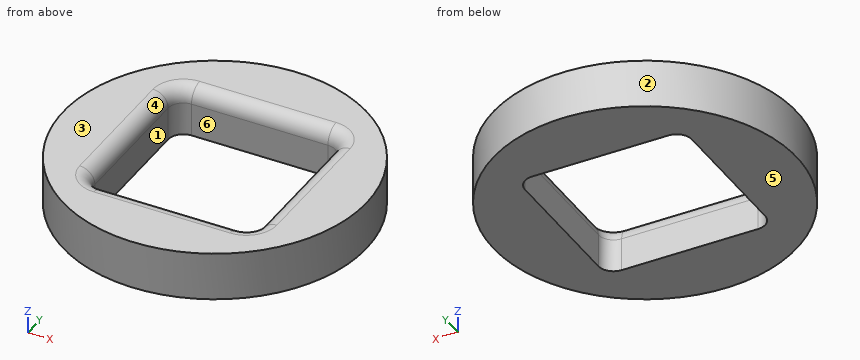
from build123d import *

# Parameters (mm, degrees)
SKETCH1_R               = 25
SKETCH1_W               = 27.5
SKETCH1_H               = 27.5
BOSS_EXTRUDE1_DEPTH     = 55
BOSS_EXTRUDE2_START     = 5
SKETCH2_R               = 25
SKETCH2_W               = 27.5
SKETCH2_H               = 27.5
BOSS_EXTRUDE2_DEPTH     = 5
SKETCH3_W               = 25
SKETCH3_H               = 50
BOSS_EXTRUDE3_DEPTH     = 80
FILLET1_R               = 2.5
FILLET2_R               = 2.5
SKETCH21_W              = 54.3
SKETCH21_H              = 20.3
CUT_EXTRUDE1_DEPTH      = 11.3
SKETCH22_W              = 40.3
SKETCH22_H              = 20.3
CUT_EXTRUDE2_DEPTH      = 93.059763198
CUT_EXTRUDE3_DEPTH      = 88.464278423
SKETCH23_R              = 2.15
CUT_EXTRUDE4_DEPTH      = 93.059763198
CUT_EXTRUDE7_DEPTH      = 27.5
CUT_EXTRUDE8_DEPTH      = 93.059763198
CUT_EXTRUDE8_DEPTH_BACK = 93.059763198
SKETCH25_W              = 132
SKETCH25_H              = 50


with BuildPart() as part:
    # Sketch1 → Boss-Extrude1 (new body)
    with BuildSketch(Plane.XY):
        Circle(SKETCH1_R)
        Rectangle(SKETCH1_W, SKETCH1_H, mode=Mode.SUBTRACT)
    extrude(amount=BOSS_EXTRUDE1_DEPTH)

    # Sketch2 → Boss-Extrude2 (add)
    # profile 1 of 2: a face of its own
    with BuildSketch(Plane(origin=(0, 0, 0), x_dir=(-1, 0, 0), z_dir=(0, 0, -1)).offset(BOSS_EXTRUDE2_START)):
        Circle(SKETCH2_R)
        Rectangle(SKETCH2_W, SKETCH2_H, mode=Mode.SUBTRACT)
    # profile 2 of 2: a face of its own
    with BuildSketch(Plane(origin=(0, 0, 0), x_dir=(-1, 0, 0), z_dir=(0, 0, -1)).offset(BOSS_EXTRUDE2_START)):
        Rectangle(SKETCH2_W, SKETCH2_H)
    extrude(amount=-BOSS_EXTRUDE2_DEPTH)

    # Sketch3 → Boss-Extrude3 (add)
    with BuildSketch(Plane(origin=(0, 0, -5), x_dir=(-1, 0, 0), z_dir=(0, 0, -1))):
        with Locations((12.5, 0)):
            Rectangle(SKETCH3_W, SKETCH3_H)
    extrude(amount=BOSS_EXTRUDE3_DEPTH)

    # Fillet1
    fillet1_edges = [part.edges().sort_by_distance(p)[0] for p in [
        (-13.75, 13.75, 27.5),
        (-13.75, -13.75, 27.5),
        (13.75, -13.75, 27.5),
        (13.75, 13.75, 27.5),
    ]]
    fillet(fillet1_edges, radius=FILLET1_R)

    # Fillet2
    fillet2_edges = [part.edges().sort_by_distance(p)[0] for p in [
        (0, 13.75, 55),
        (-13.75, 0, 55),
        (0, -13.75, 55),
        (13.75, 0, 55),
        (-13.017766953, 13.017766953, 55),
        (-13.017766953, -13.017766953, 55),
        (13.017766953, -13.017766953, 55),
        (13.017766953, 13.017766953, 55),
    ]]
    fillet(fillet2_edges, radius=FILLET2_R)

    # Sketch21 → Cut-Extrude1 (cut)
    with BuildSketch(Plane(origin=(0, 0, 0), x_dir=(0, 0, -1), z_dir=(1, 0, 0))):
        with Locations((51.85, 0)):
            Rectangle(SKETCH21_W, SKETCH21_H)
    extrude(amount=-CUT_EXTRUDE1_DEPTH, mode=Mode.SUBTRACT)

    # Sketch22 → Cut-Extrude2 (cut, through all)
    with BuildSketch(Plane(origin=(0, 0, 0), x_dir=(0, 0, -1), z_dir=(1, 0, 0))):
        with Locations((51.7, 0)):
            Rectangle(SKETCH22_W, SKETCH22_H)
    extrude(amount=-CUT_EXTRUDE2_DEPTH, mode=Mode.SUBTRACT)

    # Sketch18 → Cut-Extrude3 (cut, through all)
    with BuildSketch(Plane.XY.offset(-5)):
        with BuildLine():
            Line((-25, -25), (0, -25))
            ThreePointArc((0, -25), (-17.67766953, -17.67766953), (-25, 0))
            Line((-25, 0), (-25, -25))
        make_face()
        with BuildLine():
            Line((-25, 25), (-25, 0))
            ThreePointArc((-25, 0), (-17.67766953, 17.67766953), (0, 25))
            Line((0, 25), (-25, 25))
        make_face()
    extrude(amount=-CUT_EXTRUDE3_DEPTH, mode=Mode.SUBTRACT)

    # Sketch23 → Cut-Extrude4 (cut, through all)
    with BuildSketch(Plane(origin=(0, 0, 0), x_dir=(0, 0, -1), z_dir=(1, 0, 0))):
        with Locations(Location((27.85, -5.25, 0), (0, 0, 90))):
            Circle(SKETCH23_R)
        with Locations(Location((75.85, 5.25, 0), (0, 0, 90))):
            Circle(SKETCH23_R)
        with Locations(Location((75.85, -5.25, 0), (0, 0, 90))):
            Circle(SKETCH23_R)
        with Locations(Location((27.85, 5.25, 0), (0, 0, 90))):
            Circle(SKETCH23_R)
    extrude(amount=-CUT_EXTRUDE4_DEPTH, mode=Mode.SUBTRACT)

    # Sketch24 → Cut-Extrude7 (cut, symmetric)
    with BuildSketch(Plane(origin=(0, 0, -51.7), x_dir=(-1, 0, 0), z_dir=(0, 0, -1))):
        with BuildLine():
            Line((13.3, 10.15), (13.3, -10.15))
            Line((13.3, -10.15), (22.846826913, -10.15))
            ThreePointArc((22.846826913, -10.15), (25, 0), (22.846826913, 10.15))
            Line((22.846826913, 10.15), (13.3, 10.15))
        make_face()
    extrude(amount=CUT_EXTRUDE7_DEPTH, both=True, mode=Mode.SUBTRACT)

    # Sketch25 → Cut-Extrude8 (cut, two sides: drawn at the far end of the back side and taken through both)
    with BuildSketch(Plane(origin=(0, 0, 0), x_dir=(0, 0, -1), z_dir=(1, 0, 0)).offset(-CUT_EXTRUDE8_DEPTH_BACK)):
        with Locations((19, 0)):
            Rectangle(SKETCH25_W, SKETCH25_H)
    extrude(amount=CUT_EXTRUDE8_DEPTH + CUT_EXTRUDE8_DEPTH_BACK, mode=Mode.SUBTRACT)


solid = part.part
Build history of the part. All positions in model axes, mm. Face numbers are marked on the shaded views. A direction names the side the tool comes from. Round coordinates to 2 decimals unless told otherwise and drop trailing zeros. Loops run counter-clockwise (first coordinate to the right, second up) from the corner with the lowest first, then second, coordinate; pieces in that order, holes last. Notation, with made-up numbers: (36, 78.25) -> (85, 78.25) arc R21 cw to (85, 104.25) -> close; hole circle Ø2 at (73.5, 34). An arc over 180 degrees is marked (long way). One line per item, written item: value. Start each with the question number.
Q1. Cut at D-D on z = 51.25. List the corners of the cut face in (x, y).
Q2. Two-plate mould, pull along Y, no slides. Class the marked faces 1, 2 and 3: released by +Y, released by -Y, zero draft, split by the parting line, or undercut.
Q3. Drop flat-ended pins along their axis: pin 1 Ø4.5 at (x, z) = (1.5, 48.5) entering from +Y; pin 2 Ø3 at (y, z) = (-3.5, 51) entering from +X. Give the stop position or say it passes through.
Q4. Cut at C-C on y = 0. List the corners of the cut face in (x, z).
Q5. 3-axis set-ups, long thin cutter, end or side, ignore diameter. For the marked faces 4, 5 and 6: which of +Z, -Z, +X, -X, +Y, -Y reach the whole face in a straight line?
Q6. Cut at B-B on z = 54. List the corners of the cut face in (x, y), plus the area to 3 significant figures.
Q7. Cut at A-A on x = -7. List the corners of the cut face in (y, z), plus the area to 3 significant figures.
Q8. Probe line 1 along Z through (x, y) = (-6, -16); line 2 along X through (y, z) = (4, 52.75); line 3 along Y through (x, z) = (-4.5, 54). List the from-to ranges inside material, lowest first.
Computed:
1. outline: circle Ø50 at (0, 0); hole (-13.75, -11.25) arc R2.5 ccw to (-11.25, -13.75) -> (11.25, -13.75) arc R2.5 ccw to (13.75, -11.25) -> (13.75, 11.25) arc R2.5 ccw to (11.25, 13.75) -> (-11.25, 13.75) arc R2.5 ccw to (-13.75, 11.25) -> close
2. face 1: undercut
2. face 2: split by the parting line
2. face 3: zero draft
3. pin 1: y = 25
3. pin 2: x = 24.92
4. outline: (-25, 47) -> (-13.75, 47) -> (-13.75, 52.5) arc R2.5 ccw to (-16.25, 55) -> (-25, 55) -> close; (13.75, 47) -> (25, 47) -> (25, 55) -> (16.25, 55) arc R2.5 ccw to (13.75, 52.5) -> close
5. face 4: +Z
5. face 5: -Z, +X, -X, +Y, -Y
5. face 6: +Z, -Z
6. outline: circle Ø50 at (0, 0); hole (-14.25, -11.25) arc R3 ccw to (-11.25, -14.25) -> (11.25, -14.25) arc R3 ccw to (14.25, -11.25) -> (14.25, 11.25) arc R3 ccw to (11.25, 14.25) -> (-11.25, 14.25) arc R3 ccw to (-14.25, 11.25) -> close
6. area: 1,160 mm²
7. outline: (-24, 47) -> (-13.75, 47) -> (-13.75, 52.5) arc R2.5 ccw to (-16.25, 55) -> (-24, 55) -> close; (13.75, 47) -> (24, 47) -> (24, 55) -> (16.25, 55) arc R2.5 ccw to (13.75, 52.5) -> close
7. area: 161 mm²
8. line 1: 47 to 54.99
8. line 2: -24.68 to -13.76, 13.76 to 24.68
8. line 3: -24.59 to -14.25, 14.25 to 24.59
